Geometry check sheet. Reference: the model listing, model coordinates, mm. Face numbers are marked on the shaded views. Give positions to 0.01 mm unless a question says otherwise; leave off trailing zeros.
Autodesk Inventor part; units mm, degrees
ref_plane "YZ Plane" through (0, 0, 0) normal (1, 0, 0) x (0, 1, 0)
ref_plane "XZ Plane" through (0, 0, 0) normal (0, 1, 0) x (-1, 0, 0)
ref_plane "XY Plane" through (0, 0, 0) normal (0, 0, 1) x (1, 0, 0)
sketch "Sketch1" plane through (0, 0, 0) normal (0, 1, 0) x (-1, 0, 0)
  line L0 (0, 0) -> (-16.25, 0)
  line L1 (0, 0) -> (46.75, 0)
  line L2 (300, 0) -> (330, 0)
  line L3 (330, 30) -> (-30, 30)
  line L4 (-19.25, 8.5) -> (49.75, 8.5) construction
  line L5 (49.75, 8.5) -> (49.75, -8.5) construction
  line L6 (49.75, -8.5) -> (-19.25, -8.5) construction
  line L7 (-19.25, -8.5) -> (-19.25, 8.5) construction
  line L8 (-19.25, 8.5) -> (49.75, -8.5) construction
  line L9 (49.75, 8.5) -> (-19.25, -8.5) construction
  line L10 (-30, 0) -> (-30, 30)
  line L11 (330, 0) -> (330, 30)
  line L12 (46.75, 0) -> (300, 0)
  line L13 (-16.25, 0) -> (-30, 0)
  line L14 (0, 0) -> (-30, 0) construction
  point P0 (15.25, 0)
  point P1 (15.25, 0)
  dimension "d0" = 300
  dimension "d7" = 69
  dimension "d8" = 17
  dimension "d10" = 30
  dimension "d11" = 30
  dimension "d29" = 19.25
extrude "Extrusion1" add sketch "Sketch1" along normal blind 6
hole "Hole1" at (19.25, 0, 8.5) at (-49.75, 0, 8.5) direction (0, 1, 0) diameter 2 end through all
hole "Hole2" at (-300, 0, 0) direction (0, 1, 0) diameter 3 end through all
fillet "Fillet1" radius 20 1 edges at (30, 3, 30)
mirror "Mirror1" about plane through (16.25, 0, 0) normal (0, 0, -1)
properties part number "segment1b" material "Plywood, Finish"
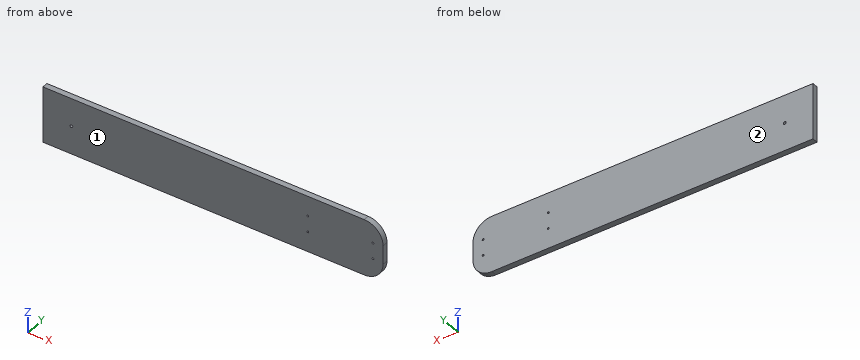
Q1. Thickness scan on L1, parallel to X at y = 2.5, z = -8.5; L2, parallel to Z at x = -49.75, y = 2.9; L3, parallel to Z at x = -300, y = 2.6. Record the ranges inside material, lowest first.
Q2. Gauge pin test, flat end, axial feed: P1, Ø1.2, axis at x = -49.75, z = -8.5, coming from the +Y side. Record the tip position at first contact, or that the pin passes through.
Q3. Release check for a two-part mould opening along Y. For the marked faces 1 and 2 record: pulls with the +Y half, pulls with the -Y half, needs draft (parallel to the pull), parting line crosses it, or undercut.
Answers follow:
1. L1: x = -330 to -50.75, -48.75 to 18.25, 20.25 to 30
1. L2: z = -30 to -9.5, -7.5 to 7.5, 9.5 to 30
1. L3: z = -30 to -1.5, 1.5 to 30
2. P1: passes through
3. face 1: pulls with the -Y half
3. face 2: pulls with the +Y half
